```python
from build123d import *

# Parameters (mm, degrees)
SKETCH_1_W          = 10
SKETCH_1_H          = 10
SKETCH_1_W_2        = 8
SKETCH_1_H_2        = 8
EXTRUDE_1_DEPTH     = 208
SKETCH_2_R          = 1.6
CUT_EXTRUDE_1_DEPTH = 209.300264042
SKETCH_3_R          = 1.6
CUT_EXTRUDE_2_DEPTH = 209.300264042
SKETCH_4_R          = 1.6
CUT_EXTRUDE_3_DEPTH = 209.300264042


with BuildPart() as part:
    # ｽｹｯﾁ1 → ﾎﾞｽ - 押し出し1 (new body)
    with BuildSketch(Plane.XY):
        Rectangle(SKETCH_1_W, SKETCH_1_H)
        Rectangle(SKETCH_1_W_2, SKETCH_1_H_2, mode=Mode.SUBTRACT)
    extrude(amount=EXTRUDE_1_DEPTH)

    # ｽｹｯﾁ2 → ｶｯﾄ - 押し出し1 (cut, through all)
    with BuildSketch(Plane(origin=(5, 0, 0), x_dir=(0, 0, -1), z_dir=(1, 0, 0))):
        with Locations(Location((-203, 0, 0), (0, 0, 90))):
            Circle(SKETCH_2_R)
        with Locations(Location((-111.5, 0, 0), (0, 0, 90))):
            Circle(SKETCH_2_R)
        with Locations(Location((-96.5, 0, 0), (0, 0, 90))):
            Circle(SKETCH_2_R)
        with Locations(Location((-5, 0, 0), (0, 0, 90))):
            Circle(SKETCH_2_R)
    extrude(amount=-CUT_EXTRUDE_1_DEPTH, mode=Mode.SUBTRACT)

    # ｽｹｯﾁ3 → ｶｯﾄ - 押し出し2 (cut, through all)
    with BuildSketch(Plane(origin=(0, 5, 0), x_dir=(1, 0, 0), z_dir=(0, 1, 0))):
        with Locations(Location((0, -193, 0), (0, 0, 270))):
            Circle(SKETCH_3_R)
        with Locations(Location((0, -15, 0), (0, 0, 270))):
            Circle(SKETCH_3_R)
    extrude(amount=-CUT_EXTRUDE_2_DEPTH, mode=Mode.SUBTRACT)

    # ｽｹｯﾁ4 → ｶｯﾄ - 押し出し3 (cut, through all)
    with BuildSketch(Plane(origin=(5, 0, 0), x_dir=(0, 0, -1), z_dir=(1, 0, 0))):
        with Locations(Location((-129, 0, 0), (0, 0, 90))):
            Circle(SKETCH_4_R)
        with Locations(Location((-79, 0, 0), (0, 0, 90))):
            Circle(SKETCH_4_R)
    extrude(amount=-CUT_EXTRUDE_3_DEPTH, mode=Mode.SUBTRACT)


solid = part.part
```
Design review of the part built by this model. Coordinates are the model's own, in mm. A direction names the side the tool comes from. Give positions to 0.01 mm unless a question says otherwise; leave off trailing zeros. Loops run counter-clockwise (first coordinate to the right, second up) from the corner with the lowest first, then second, coordinate; pieces in that order, holes last. Notation, with made-up numbers: M 75.5,4 L 89.5,4 A17 cw 89.5,31 Z; hole C 11,-3.5 d1. An arc over 180 degrees is marked long. Return JSON: item names as keys, results as strings. Group by question number.
Item 1: Tool access review of faces 1 (the cylindrical face through (-4.493, -0.208, 113.086)), 2 (the flat face through (0, 4, 103)): name each direction out of +Z, -Z, +X, -X, +Y, -Y from which nothing blocks a thin tool from reaching the whole face with its end or side.
Item 2: We need section C-C (y = 0). Give the number of separate pieces and of enclosed holes in the cut face, and give its area (3 significant figures).
Item 3: Insertion check: pin 1 Ø1.9 at (y, z) = (0, 203) entering from +X. The pin has a flat end and moves straight along its axis. Give the tip position at first contact, or say it passes through.
Item 4: We need section B-B (x = 0). Give the boundary of the cut face in (y, z).
Item 5: Mouldability with a two-part tool opening along X and no side actions: class faces 3 (the cylindrical face through (4.507, -0.208, 113.086)), 4 (the flat face through (-5, 0, 103)), 5 (the cylindrical face through (-0.61, -4.49, 194.48)), 6 (the flat face through (5, 0, 103)) as released by +X, released by -X, zero draft, split by the parting line, or undercut.
Item 6: We need section A-A (z = 168). Give the boundary of the cut face in (x, y), and give its area (3 significant figures).
Item 7: For probe 1 along X at (y, z) = (-2, 126); probe 2 along Y at (x, z) = (-4.4, 79), list the stretches that pass through material, from the lowest coordinate up.
Output:
{
 "1": {"face 1": "+X, -X", "face 2": "+Z, -Z"},
 "2": {"separate pieces": "14", "enclosed holes": "0", "area": "378 mm^2"},
 "3": {"pin 1": "passes through"},
 "4": {"outline": "M -5,0 L -4,0 L -4,13.4 L -5,13.4 Z; M -5,16.6 L -4,16.6 L -4,191.4 L -5,191.4 Z; M -5,194.6 L -4,194.6 L -4,208 L -5,208 Z; M 4,0 L 5,0 L 5,13.4 L 4,13.4 Z; M 4,16.6 L 5,16.6 L 5,191.4 L 4,191.4 Z; M 4,194.6 L 5,194.6 L 5,208 L 4,208 Z"},
 "5": {"face 3": "zero draft", "face 4": "released by -X", "face 5": "undercut", "face 6": "released by +X"},
 "6": {"outline": "M -5,-5 L 5,-5 L 5,5 L -5,5 Z; hole M -4,-4 L 4,-4 L 4,4 L -4,4 Z", "area": "36.0 mm^2"},
 "7": {"probe 1": "x = -5 to -4, 4 to 5", "probe 2": "y = -5 to -1.6, 1.6 to 5"}
}
